The listing builds one solid part. Answer for the finished solid, in the listing's coordinates (mm). A direction names the side the tool comes from. Round coordinates to 2 decimals unless told otherwise and drop trailing zeros. Write each loop counter-clockwise with the first axis right and the second up, starting at its lowest first coordinate (ties: lowest second). Pieces come first, ordered by that corner, then holes.
(1) A cutting plane is placed at B-B, the plane y = 54. Give the vertices of the cut face in (x, z).
(2) Find the intervals of material crossed by probe 1 along Y at (x, z) = (-10, 1.1); probe 2 along X at (y, z) = (80.5, 1.15); probe 3 along Y at (x, z) = (-4.25, 2.7), in increasing order.
(3) A cutting plane is placed at C-C, the plane x = -13.75. Give the vertices of the cut face in (y, z), and give its area (3 significant figures).
(4) For faces 1 (the face through (-17.93, 39.1, 1.52)), 2 (the face through (-20, 43, 1)), determine the directions among +Z, -Z, +X, -X, +Y, -Y from which every point of the face is accessible in a straight line to the end or side of a thin tool.
(5) The mould has two halves that part along Y. Classify faces 3 (the face through (-19, 43, 3)), 4 (the face through (-2.07, 39.1, 1.52)), 5 (the face through (-0.6, 0.57, 1.52)): +Y half, -Y half, draft (parallel to the pull), parting line (faces both ways), or undercut.
(6) A cutting plane is placed at A-A, the plane x = -10. Give the vertices of the cut face in (y, z), and give its area (3 significant figures).
from build123d import *

# Parameters (mm, degrees)
SKETCH_1_W      = 88
SKETCH_1_H      = 20
SKETCH_1_R      = 2.4
SKETCH_1_R_2    = 1.55
SKETCH_1_W_2    = 11
SKETCH_1_H_2    = 17
EXTRUDE_1_DEPTH = 3
FILLET_1_R      = 2


with BuildPart() as part:
    # ｽｹｯﾁ1 → ﾎﾞｽ - 押し出し1 (new body)
    with BuildSketch(Plane(origin=(0, 0, 0), x_dir=(0, 1, 0), z_dir=(0, 0, 1))):
        with Locations((44, 10)):
            Rectangle(SKETCH_1_W, SKETCH_1_H)
        with Locations((7.5, 10)):
            Circle(SKETCH_1_R, mode=Mode.SUBTRACT)
        with Locations((80.5, 10)):
            Circle(SKETCH_1_R, mode=Mode.SUBTRACT)
        with Locations((54, 10)):
            Circle(SKETCH_1_R_2, mode=Mode.SUBTRACT)
        with Locations((34, 10)):
            Circle(SKETCH_1_R_2, mode=Mode.SUBTRACT)
        with Locations((44, 10)):
            Rectangle(SKETCH_1_W_2, SKETCH_1_H_2, mode=Mode.SUBTRACT)
    extrude(amount=EXTRUDE_1_DEPTH)

    # ﾌｨﾚｯﾄ1
    fillet_1_edges = [part.edges().sort_by_distance(p)[0] for p in [
        (-1.5, 49.5, 1.5),
        (-18.5, 49.5, 1.5),
        (-18.5, 38.5, 1.5),
        (-1.5, 38.5, 1.5),
        (-20, 0, 1.5),
        (-20, 88, 1.5),
        (0, 88, 1.5),
        (0, 0, 1.5),
    ]]
    fillet(fillet_1_edges, radius=FILLET_1_R)


solid = part.part
Solutions:
1. outline: (-20, 0) - (-11.55, 0) - (-11.55, 3) - (-20, 3) - close; (-8.45, 0) - (0, 0) - (0, 3) - (-8.45, 3) - close
2. probe 1: y = 0 to 5.1, 9.9 to 32.45, 35.55 to 38.5, 49.5 to 52.45, 55.55 to 78.1, 82.9 to 88
2. probe 2: x = -20 to -12.4, -7.6 to 0
2. probe 3: y = 0 to 38.5, 49.5 to 88
3. outline: (0, 0) - (38.5, 0) - (38.5, 3) - (0, 3) - close; (49.5, 0) - (88, 0) - (88, 3) - (49.5, 3) - close
3. area: 231 mm2
4. face 1: +Z, -Z
4. face 2: +Z, -Z, -X, +Y, -Y
5. face 3: draft
5. face 4: undercut
5. face 5: -Y half
6. outline: (0, 0) - (5.1, 0) - (5.1, 3) - (0, 3) - close; (9.9, 0) - (32.45, 0) - (32.45, 3) - (9.9, 3) - close; (35.55, 0) - (38.5, 0) - (38.5, 3) - (35.55, 3) - close; (49.5, 0) - (52.45, 0) - (52.45, 3) - (49.5, 3) - close; (55.55, 0) - (78.1, 0) - (78.1, 3) - (55.55, 3) - close; (82.9, 0) - (88, 0) - (88, 3) - (82.9, 3) - close
6. area: 184 mm2
